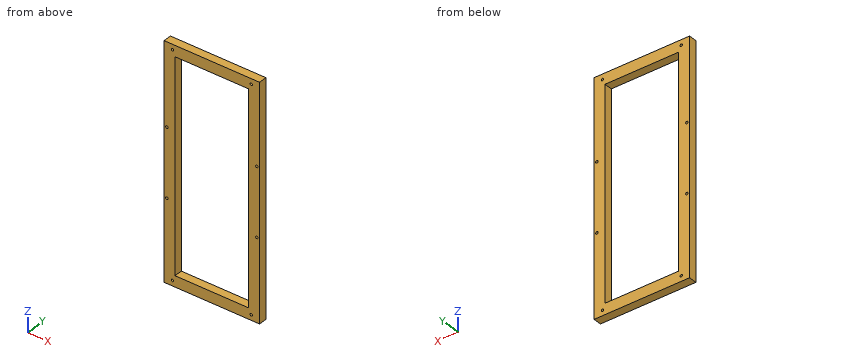
Autodesk Inventor part; units mm, degrees
ref_plane "YZ Plane" through (0, 0, 0) normal (1, 0, 0) x (0, 1, 0)
ref_plane "XZ Plane" through (0, 0, 0) normal (0, 1, 0) x (-1, 0, 0)
ref_plane "XY Plane" through (0, 0, 0) normal (0, 0, 1) x (1, 0, 0)
sketch "Sketch1" plane through (0, 0, 0) normal (0, 1, 0) x (-1, 0, 0)
  line L0 (-27, 77) -> (27, 77)
  line L1 (27, 77) -> (27, -77)
  line L2 (27, -77) -> (-27, -77)
  line L3 (-27, -77) -> (-27, 77)
  line L4 (-27, 77) -> (27, -77) construction
  line L5 (27, 77) -> (-27, -77) construction
  line L6 (-35, 85) -> (35, 85)
  line L7 (35, 85) -> (35, -85)
  line L8 (35, -85) -> (-35, -85)
  line L9 (-35, -85) -> (-35, 85)
  line L10 (-35, 85) -> (35, -85) construction
  line L11 (35, 85) -> (-35, -85) construction
  circle A0 centre (28.875, -81.087) radius 0.9
  circle A1 centre (33, -25) radius 0.9
  line L12 (0, 0) -> (0, -26.4871)
  line L13 (0, 0) -> (15.9434, 0)
  circle A2 centre (-28.875, -81.087) radius 0.9
  circle A3 centre (-33, -25) radius 0.9
  circle A4 centre (28.875, 81.087) radius 0.9
  circle A5 centre (33, 25) radius 0.9
  circle A6 centre (-28.875, 81.087) radius 0.9
  circle A7 centre (-33, 25) radius 0.9
  dimension "d0" = 8
  dimension "d1" = 8
  dimension "d2" = 70
  dimension "d3" = 170
  dimension "d6" = 1.8
  dimension "d7" = 1.8
  dimension "d8" = 57.75
  dimension "d9" = 33
  dimension "d10" = 25
extrude "Extrusion1" add sketch "Sketch1" along normal blind 6
equation "\"d1\" = d0"
properties part number "case_top_cover_slot" material "Acrylic, Clear"
The listing builds one solid part. Answer for the finished solid, in the listing's coordinates (mm). Coordinates: 2 decimals unless noted, no trailing zeros. Write each loop counter-clockwise with the first axis right and the second up, starting at its lowest first coordinate (ties: lowest second). Pieces come first, ordered by that corner, then holes. Notation, with made-up numbers: M -28.5,-32.5 L -15.5,-32.5 A20 ccw -15.5,-0.5 Z; hole C -29.5,52.5 d10. An arc over 180 degrees is marked long. Write each question's results on one line, items separated by ' | '.
Item 1: The part is cut by section C-C on y = 4.8. State how many separate pieces and enclosed holes the cut face has, and give its area (3 significant figures).
Answer below:
separate pieces: 1 | enclosed holes: 9 | area: 3,560 mm2
Item 2: Given P1, Ø3, axis at x = 28.875, z = -81.087, coming from the -Y side; P2, Ø1.4, axis at x = -33, z = -25, coming from the +Y side, each flat-ended and moving along its own axis, determine where each tip first touches the part or whether it passes through.
Answer below:
P1: y = 0 | P2: through
Item 3: The part is cut by section A-A on z = -38.5. Determine the outline of the cut face in (x, y).
Answer below:
outline: M -35,0 L -27,0 L -27,6 L -35,6 Z; M 27,0 L 35,0 L 35,6 L 27,6 Z
Item 4: The part is cut by section B-B on x = -9. Determine the outline of the cut face in (y, z).
Answer below:
outline: M 0,-85 L 6,-85 L 6,-77 L 0,-77 Z; M 0,77 L 6,77 L 6,85 L 0,85 Z
Item 5: Consider probe 1 along Z at (x, y) = (33, 2.4); probe 2 along X at (y, z) = (2.3, -65); probe 3 along Z at (x, y) = (5.5, 4.05). Determine where each line is inside the solid, lowest interval first. Write a range as [from, to].
Answer below:
probe 1: [-85, -25.9], [-24.1, 24.1], [25.9, 85] | probe 2: [-35, -27], [27, 35] | probe 3: [-85, -77], [77, 85]
